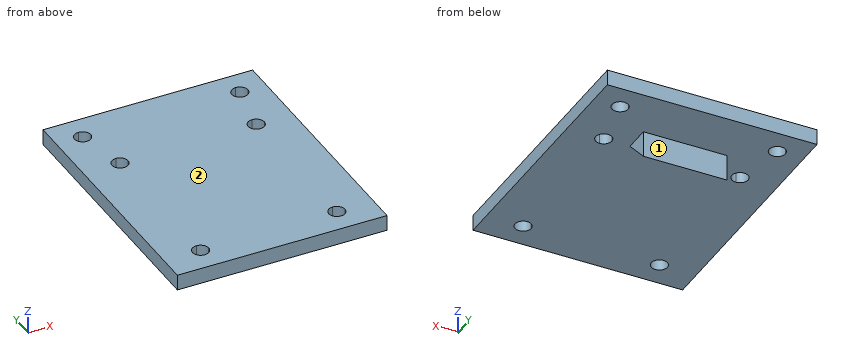
```python
from build123d import *

# Parameters (mm, degrees)
F0_W     = 16
F0_H     = 5
F1_DEPTH = 3
F2_DEPTH = 5
F3_SIZE  = 4.99999


# Not quite as in the source:
# - a fillet or chamfer is up to 0.001 mm smaller than in the source, because OpenCascade refuses the exact size


with BuildPart() as f1:
    # F0 (on Top) → F1 (new body)
    with BuildSketch(Plane.XY):
        with BuildLine():
            ThreePointArc((-13, -13.45), (-11.9039844892, -13.9039844892), (-11.45, -15))
            Line((-11.45, -15), (11.45, -15))
            ThreePointArc((11.45, -15), (11.9039844892, -13.9039844892), (13, -13.45))
            Line((13, -13.45), (13, 13.45))
            ThreePointArc((13, 13.45), (11.9039844892, 13.9039844892), (11.45, 15))
            Line((11.45, 15), (8, 15))
            Line((8, 15), (-8, 15))
            Line((-8, 15), (-11.45, 15))
            ThreePointArc((-11.45, 15), (-11.9039844892, 13.9039844892), (-13, 13.45))
            Line((-13, 13.45), (-13, -13.45))
        make_face()
        with BuildLine():
            Line((11.45, -15), (-11.45, -15))
            ThreePointArc((-11.45, -15), (-14.0960155108, -16.0960155108), (-13, -13.45))
            Line((-13, -13.45), (-13, 13.45))
            ThreePointArc((-13, 13.45), (-14.55, 15), (-13, 16.55))
            Line((-13, 16.55), (-13, 20))
            Line((-13, 20), (-20, 20))
            Line((-20, 20), (-20, -20))
            Line((-20, -20), (20, -20))
            Line((20, -20), (20, 20))
            Line((20, 20), (13, 20))
            Line((13, 20), (13, 16.55))
            ThreePointArc((13, 16.55), (14.0960155108, 16.0960155108), (14.55, 15))
            ThreePointArc((14.55, 15), (14.0960155108, 13.9039844892), (13, 13.45))
            Line((13, 13.45), (13, -13.45))
            ThreePointArc((13, -13.45), (14.0960155108, -13.9039844892), (14.55, -15))
            ThreePointArc((14.55, -15), (13, -16.55), (11.45, -15))
        make_face()
        with BuildLine():
            Line((-13, 20), (-13, 16.55))
            ThreePointArc((-13, 16.55), (-11.9039844892, 16.0960155108), (-11.45, 15))
            Line((-11.45, 15), (-8, 15))
            Line((-8, 15), (-8, 20))
            Line((-8, 20), (-13, 20))
        make_face()
        with BuildLine():
            Line((8, 15), (11.45, 15))
            ThreePointArc((11.45, 15), (11.9039844892, 16.0960155108), (13, 16.55))
            Line((13, 16.55), (13, 20))
            Line((13, 20), (8, 20))
            Line((8, 20), (8, 15))
        make_face()
        with BuildLine():
            Line((-20, 20), (-13, 20))
            Line((-13, 20), (-8, 20))
            Line((-8, 20), (8, 20))
            Line((8, 20), (13, 20))
            Line((13, 20), (20, 20))
            Line((20, 20), (20, 30))
            Line((20, 30), (15, 30))
            Line((15, 30), (15, 26.55))
            ThreePointArc((15, 26.55), (16.0960155108, 26.0960155108), (16.55, 25))
            ThreePointArc((16.55, 25), (15, 23.45), (13.45, 25))
            Line((13.45, 25), (-13.45, 25))
            ThreePointArc((-13.45, 25), (-15, 23.45), (-16.55, 25))
            Line((-16.55, 25), (-20, 25))
            Line((-20, 25), (-20, 20))
        make_face()
        with Locations((0, 17.5)):
            Rectangle(F0_W, F0_H)
        with BuildLine():
            Line((-20, 30), (-20, 25))
            Line((-20, 25), (-16.55, 25))
            ThreePointArc((-16.55, 25), (-16.0960155108, 26.0960155108), (-15, 26.55))
            Line((-15, 26.55), (-15, 30))
            Line((-15, 30), (-20, 30))
        make_face()
        with BuildLine():
            Line((15, 30), (-15, 30))
            Line((-15, 30), (-15, 26.55))
            ThreePointArc((-15, 26.55), (-13.9039844892, 26.0960155108), (-13.45, 25))
            Line((-13.45, 25), (13.45, 25))
            ThreePointArc((13.45, 25), (13.9039844892, 26.0960155108), (15, 26.55))
            Line((15, 26.55), (15, 30))
        make_face()
    extrude(amount=F1_DEPTH)

    # F0 (on Top) → F2 (join)
    with BuildSketch(Plane.XY):
        with Locations((0, 17.5)):
            Rectangle(F0_W, F0_H)
    extrude(amount=-F2_DEPTH)

    # F3 (size 5 in the source; OpenCascade refuses exactly that, so slightly less here)
    f3_edges = [f1.edges().sort_by_distance(p)[0] for p in [
        (0, 15, -5),
    ]]
    chamfer(f3_edges, length=F3_SIZE)


solid = f1.part
```
Source: CAD feature listing. Evaluate the final solid. Frame: model axes, mm. Face numbers are marked on the shaded views. A direction names the side the tool comes from. Round coordinates to 2 decimals unless told otherwise and drop trailing zeros. Write each loop counter-clockwise with the first axis right and the second up, starting at its lowest first coordinate (ties: lowest second). Pieces come first, ordered by that corner, then holes. Notation, with made-up numbers: M 30,62.25 L 73,62.25 A27 cw 73,97.25 Z; hole C -19,-18 d1. An arc over 180 degrees is marked long. Use CSV: the item, a comma, the result in double quotes. Start each with the question number.
Q1. Cut plane C-C on y = 6.5. Output: boundary loops of the cut face in (x, z), plus the area to 3 significant figures.
Q2. Cut plane A-A on x = -16. Output: boundary loops of the cut face in (y, z), plus the area to 3 significant figures.
Q3. Line query: line 1 (Y direction, x = -13, z = 1.4); line 2 (X direction, y = -15, z = 1.25); line 3 (Z direction, x = 15.5, y = -1.5). Output: solid intervals per line, ascending. Write a range as from..to.
Q4. Access query for the marked faces 1 and 2. Directions: +Z, -Z, +X, -X, +Y, -Y. A direction counts if a zero-diameter tool reaches every point of the face in a straight line with its end or side. Return the directions, or none.
Q5. First-contact query: P1, Ø2.5, axis at y = 16.5, z = -2.5, coming from the +X side; P2, Ø1.5, axis at y = 17, z = -1.5, coming from the -X side; P3, Ø1, axis at x = 5.5, y = 22.5, coming from the -Z side. Flat tips, straight axial feed; report the tip coordinate or a pass-through.
Q6. Cut plane D-D on z = -2.5. Output: boundary loops of the cut face in (x, y), plus the area to 3 significant figures.
Results found:
1,outline,"M -20,0 L 20,0 L 20,3 L -20,3 Z"
1,area,"120 mm^2"
2,outline,"M -20,0 L 23.82,0 L 23.82,3 L -20,3 Z; M 26.18,0 L 30,0 L 30,3 L 26.18,3 Z"
2,area,"143 mm^2"
3,line 1,"-20..-16.55, -13.45..13.45, 16.55..30"
3,line 2,"-20..-14.55, -11.45..11.45, 14.55..20"
3,line 3,"0..3"
4,face 1,"-Z, +X, -X, +Y"
4,face 2,"+Z, +X, -X, +Y, -Y"
5,P1,"x = 8"
5,P2,"x = -8"
5,P3,"z = 0"
6,outline,"M -8,17.5 L 8,17.5 L 8,20 L -8,20 Z"
6,area,"40.0 mm^2"
